```python
from build123d import *

# Parameters (mm, degrees)
SKETCH_1_W               = 70
SKETCH_1_H               = 70
SKETCH_1_W_2             = 40
SKETCH_1_H_2             = 40
EXTRUDE_1_DEPTH          = 80
SKETCH_3_W               = 40
SKETCH_3_H               = 40
EXTRUDE_2_DEPTH          = 15
SKETCH_4_R               = 2.5
CUT_EXTRUDE_1_DEPTH      = 15
SKETCH_5_R               = 30
CUT_EXTRUDE_3_DEPTH      = 70
EXTRUDE_START            = -10
EXTRUDE_4_DEPTH          = 10
SKETCH_8_W               = 19.934341116
SKETCH_8_H               = 60
CUT_EXTRUDE_6_DEPTH      = 35
SKETCH_9_W               = 15
SKETCH_9_H               = 15
EXTRUDE_5_DEPTH          = 0.001
EXTRUDE_6_DEPTH          = 50
SKETCH_11_W              = 15
SKETCH_11_H              = 15
EXTRUDE_7_DEPTH          = 10
PATTERN_CIRCULAR_1_COUNT = 4


with BuildPart() as part:
    # 草图1 → 凸台-拉伸1 (new body)
    with BuildSketch(Plane.XY):
        with Locations((7.829504232, -18.198307134)):
            Rectangle(SKETCH_1_W, SKETCH_1_H)
        with Locations((7.845306404, -19.744690932)):
            Rectangle(SKETCH_1_W_2, SKETCH_1_H_2, mode=Mode.SUBTRACT)
    extrude(amount=EXTRUDE_1_DEPTH)

    # 草图3 → 凸台-拉伸2 (add)
    with BuildSketch(Plane.XY.offset(80)):
        with Locations((7.845306404, -19.744690932)):
            Rectangle(SKETCH_3_W, SKETCH_3_H)
    extrude(amount=-EXTRUDE_2_DEPTH)

    # 草图4 → 切除-拉伸1 (cut)
    with BuildSketch(Plane.XY.offset(80)):
        with Locations((7.829504232, -18.198307134)):
            Circle(SKETCH_4_R)
    extrude(amount=-CUT_EXTRUDE_1_DEPTH, mode=Mode.SUBTRACT)

    # 草图5 → 切除-拉伸3 (cut)
    with BuildSketch(Plane(origin=(0, 0, 65), x_dir=(-1, 0, 0), z_dir=(0, 0, -1))):
        with Locations(Location((-7.829504232, -18.198307134, 0), (0, 0, 180))):
            Circle(SKETCH_5_R)
    extrude(amount=CUT_EXTRUDE_3_DEPTH, mode=Mode.SUBTRACT)

    # 草图7 → 凸台-拉伸4 (add)
    with BuildSketch(Plane(origin=(0, 0, 0), x_dir=(-1, 0, 0), z_dir=(0, 0, -1)).offset(EXTRUDE_START)):
        with BuildLine():
            Line((-17.829504232, 10.085964113), (-17.829504232, -46.482578382))
            ThreePointArc((-17.829504232, -46.482578382), (-37.829504232, -18.198307134), (-17.829504232, 10.085964113))
        make_face()
        with BuildLine():
            Line((2.170495768, 10.085964113), (2.170495768, -46.482578382))
            ThreePointArc((2.170495768, -46.482578382), (22.170495768, -18.198307134), (2.170495768, 10.085964113))
        make_face()
    extrude(amount=EXTRUDE_4_DEPTH)

    # 草图8 → 切除-拉伸6 (cut)
    with BuildSketch(Plane(origin=(0, 0, 0), x_dir=(-1, 0, 0), z_dir=(0, 0, -1))):
        with Locations((-7.862333674, -18.198307134)):
            Rectangle(SKETCH_8_W, SKETCH_8_H)
    extrude(amount=-CUT_EXTRUDE_6_DEPTH, mode=Mode.SUBTRACT)

    # 草图9 → 凸台-拉伸5 (add)
    with BuildSketch(Plane.XY.offset(80)):
        with Locations((-19.670495768, -45.698307134)):
            Rectangle(SKETCH_9_W, SKETCH_9_H)
    extrude_5 = extrude(amount=EXTRUDE_5_DEPTH)

    # 草图10 → 凸台-拉伸6 (add)
    with BuildSketch(Plane.XY.offset(80.001)):
        Polygon((-27.170495768, -38.198307134), (-19.670495768, -38.198307134), (-27.170495768, -45.698307134), align=None)
        Polygon((-19.670495768, -53.198307134), (-12.170495768, -53.198307134), (-12.170495768, -45.698307134), align=None)
    extrude_6 = extrude(amount=EXTRUDE_6_DEPTH)

    # 草图11 → 凸台-拉伸7 (add)
    with BuildSketch(Plane.XY.offset(130.001)):
        with Locations((-19.670495768, -45.698307134)):
            Rectangle(SKETCH_11_W, SKETCH_11_H)
    extrude_7 = extrude(amount=EXTRUDE_7_DEPTH)

    # 阵列(圆周)1: 凸台-拉伸5, 凸台-拉伸6, 凸台-拉伸7 ×4 about axis
    pattern_circular_1_axis = Axis((7.829504232, -18.198307134, 0), (0, 0, 1))
    add([extrude_5.rotate(pattern_circular_1_axis, i * 360 / PATTERN_CIRCULAR_1_COUNT) for i in range(1, PATTERN_CIRCULAR_1_COUNT)])
    add([extrude_6.rotate(pattern_circular_1_axis, i * 360 / PATTERN_CIRCULAR_1_COUNT) for i in range(1, PATTERN_CIRCULAR_1_COUNT)])
    add([extrude_7.rotate(pattern_circular_1_axis, i * 360 / PATTERN_CIRCULAR_1_COUNT) for i in range(1, PATTERN_CIRCULAR_1_COUNT)])


solid = part.part
```
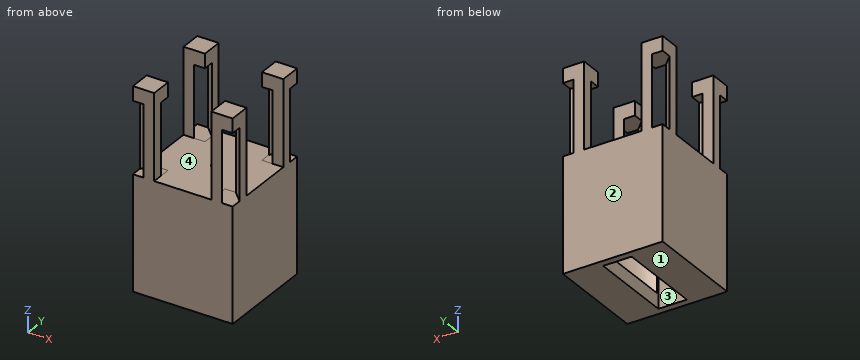
Work out the finished part from the listing and answer in its coordinate system (mm). Face numbers are marked on the shaded views. Give positions to 0.01 mm unless a question says otherwise; leave off trailing zeros. Order: outer loops, then holes, each group sorted by start corner. A loop starts at its lowest first (then second) coordinate and runs counter-clockwise, first axis right, second up. Notation, with made-up numbers: M 33.5,88.25 L 70.5,88.25 A14 ccw 70.5,108.25 Z; hole C 71,-38 d3. An arc over 180 degrees is marked long. Return JSON: item names as keys, results as strings.
1) For a pull along Y with two mould halves and no side action, classify the marked faces 1, 2, 3 and 4 as +Y half, -Y half, draft (parallel to the pull), parting line (faces both ways), or undercut.
Resolved:
{"face 1": "draft", "face 2": "+Y half", "face 3": "undercut", "face 4": "undercut"}
2) Section B-B, the plane x = 21 is taken. Write down the section's boundary in (y, z).
Resolved:
{"outline": "M -53.2,0 L 16.8,0 L 16.8,80 L -53.2,80 Z; hole M -45.15,10 L 8.76,10 L 8.76,65 L -45.15,65 Z"}
3) Section C-C, the plane y = -3.5 is taken. Write down the section's boundary in (x, z).
Resolved:
{"outline": "M -27.17,0 L -2.17,0 L -2.17,10 L -18.32,10 L -18.32,65 L 33.98,65 L 33.98,10 L 17.83,10 L 17.83,0 L 42.83,0 L 42.83,80 L -27.17,80 Z"}
4) Straight lines are drawn through the part: line 1 along Z through (x, y) = (-11.5, -33.5); line 2 along X through (y, z) = (-47, 12); line 3 along Z through (x, y) = (14, 9). For each, find the intervals that lie inside material, in ascending order. Write a range as [from, to].
Resolved:
{"line 1": "[0, 10], [65, 80]", "line 2": "[-27.17, -2.1], [17.83, 42.83]", "line 3": "[65, 80]"}
5) Section D-D, the plane x = 2 is taken. Write down the section's boundary in (y, z).
Resolved:
{"outline": "M -53.2,0 L -48.2,0 L -48.2,35 L -47.63,35 L -47.63,65 L 11.23,65 L 11.23,35 L 11.8,35 L 11.8,0 L 16.8,0 L 16.8,80 L -53.2,80 Z"}
6) Each of these flat-tipped pins is pushed along its axis until it touches: pin 1 (3 mm diameter, centred on x = 11.5, y = -11, fed in from -Z); pin 2 (1.9 mm diameter, centred on x = 2, y = -47, fed in from -Z); pin 3 (22 mm diameter, centred on x = -8, y = -12.5, fed in from +Z). Where does it stop, or does it pass through?
Resolved:
{"pin 1": "z = 65", "pin 2": "z = 35", "pin 3": "z = 80"}
7) Section A-A, the plane z = 88 is taken. Write down the section's boundary in (x, y), plus the area to 3 significant figures.
Resolved:
{"outline": "M -27.17,-45.7 L -19.67,-38.2 L -27.17,-38.2 Z; M -27.17,1.8 L -19.67,1.8 L -27.17,9.3 Z; M -19.67,-53.2 L -12.17,-53.2 L -12.17,-45.7 Z; M -19.67,16.8 L -12.17,9.3 L -12.17,16.8 Z; M 27.83,-53.2 L 35.33,-53.2 L 27.83,-45.7 Z; M 27.83,9.3 L 35.33,16.8 L 27.83,16.8 Z; M 35.33,-38.2 L 42.83,-45.7 L 42.83,-38.2 Z; M 35.33,1.8 L 42.83,1.8 L 42.83,9.3 Z", "area": "225 mm^2"}
